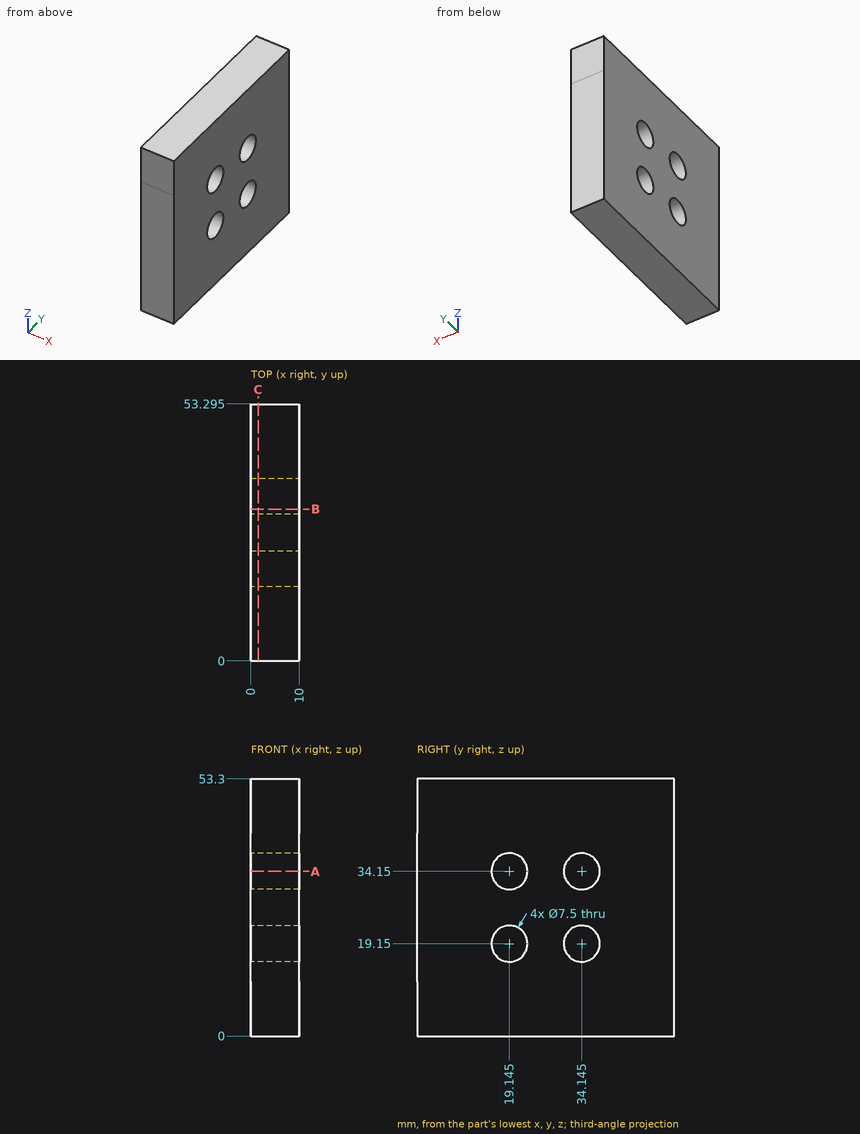
For this review, use the dimensioned drawing (mm, ordinates from the lowest corner) and the shaded views. Give positions to 0.01 mm unless a question says otherwise; leave off trailing zeros. Write each loop counter-clockwise with the first axis right and the second up, starting at its lowest first coordinate (ties: lowest second). Pieces come first, ordered by that corner, then holes. Notation, with made-up numbers: M -27,-23 L 19,-23 A25 ccw 19,12 Z; hole C 73,18 d3. An arc over 180 degrees is marked long. Write item = value, one per line. Start each with the question number.
Q1. For line 1 (Y direction, x = 5, z = 34) (1 decimal); line 2 (Z direction, x = 9, y = 36); line 3 (Y direction, x = 6.5, z = 37.5) (1 decimal), list the stretches that pass through material, from the lowest coordinate up.
Q2. Clearance check with a flat-ended pin moving along its axis: pin 1 (6 mm diameter, centred on y = 34.14, z = 34.15, fed in from +X). State where the tip first meets the part, or that it passes through.
Q3. We need section A-A (z = 34.15). State the section outline as (x, y) points (1 decimal), plus the area to 3 significant figures.
Q4. We need section C-C (x = 1.5). Give the number of separate pieces and of enclosed holes in the cut face, plus the area to 3 significant figures.
Q5. We need section B-B (y = 31.5). State the section outline as (x, z) points.
Result set:
q1.line_1 = 0 to 15.4, 22.9 to 30.4, 37.9 to 53.3
q1.line_2 = 0 to 15.89, 22.41 to 30.89, 37.41 to 53.3
q1.line_3 = 0 to 17.5, 20.8 to 32.5, 35.8 to 53.3
q2.pin_1 = through
q3.outline = M 0,0 L 10,0 L 10,15.4 L 0,15.4 Z; M 0,22.9 L 10,22.9 L 10,30.4 L 0,30.4 Z; M 0,37.9 L 10,37.9 L 10,53.3 L 0,53.3 Z
q3.area = 383 mm2
q4.separate_pieces = 1
q4.enclosed_holes = 4
q4.area = 2,660 mm2
q5.outline = M 0,0 L 10,0 L 10,16.49 L 0,16.49 Z; M 0,21.81 L 10,21.81 L 10,31.49 L 0,31.49 Z; M 0,36.81 L 10,36.81 L 10,53.3 L 0,53.3 Z
